```python
from build123d import *

# Parameters (mm, degrees)
F1_DEPTH = 5
F2_SIZE  = 2
F0_W     = 2.8
F0_H     = 9.8
F3_DEPTH = 2


# Not quite as in the source:
# - a feature of the source that left no trace in its solid (it failed there, or was rolled back) is left out


with BuildPart() as f1:
    # F0 (on Top) → F1 (new body)
    with BuildSketch(Plane.XY):
        Polygon((49.7136654785, 23.7398390386), (-80.2863345215, 29.3157004521), (-80.2863345215, 19.5157004521), (-80.2863345215, 15.7984595098), (49.7136654785, 15.7984595098), (73.3425258757, -14.2773987355), (73.3425258757, -14.4394316876), (85.7469019117, -14.4394316876), (88.3425258757, -11.6024324968), align=None)
    extrude(amount=F1_DEPTH)

    # F2 (call 1 of 5: OpenCascade refuses the feature's edges together)
    f2_edges = [f1.edges().sort_by_distance(p)[0] for p in [
        (-15.286335, 15.79846, 0),
    ]]
    chamfer(f2_edges, length=F2_SIZE)

    # F2#2 (call 2 of 5)
    f2_2_edges = [f1.edges().sort_by_distance(p)[0] for p in [
        (69.028096, 6.068703, 0),
    ]]
    chamfer(f2_2_edges, length=F2_SIZE)

    # F2#3 (call 3 of 5)
    f2_3_edges = [f1.edges().sort_by_distance(p)[0] for p in [
        (79.544714, -14.439432, 0),
    ]]
    chamfer(f2_3_edges, length=F2_SIZE)

    # F2#4 (call 4 of 5)
    f2_4_edges = [f1.edges().sort_by_distance(p)[0] for p in [
        (61.528096, 0.76053, 5),
        (-15.286335, 15.79846, 5),
    ]]
    chamfer(f2_4_edges, length=F2_SIZE)

    # F2#5 (call 5 of 5)
    f2_5_edges = [f1.edges().sort_by_distance(p)[0] for p in [
        (-15.286335, 26.52777, 5),
    ]]
    chamfer(f2_5_edges, length=F2_SIZE)

    # F0 (on Top) → F3 (join)
    with BuildSketch(Plane.XY):
        with Locations((-81.6863345215, 24.4157004521)):
            Rectangle(F0_W, F0_H)
    extrude(amount=F3_DEPTH)


solid = f1.part
```
Verification items for the finished model (mm, model axes). A direction names the side the tool comes from. Coordinates: 2 decimals unless noted, no trailing zeros. Loops run counter-clockwise (first coordinate to the right, second up) from the corner with the lowest first, then second, coordinate; pieces in that order, holes last. Notation, with made-up numbers: (-21.75, 11.25) - (-7.75, 11.25) arc R13 cw to (-7.75, 31.25) - close; hole circle Ø3 at (32.5, 88.25). An arc over 180 degrees is marked (long way). Put each result on its own line as item: value.
Item 1: Section check B-B (y = -7). Enter the section's corners in (x, z).
Conclusion:
outline: (67.63, 0) - (80.35, 0) - (83.31, 2) - (83.31, 5) - (70.17, 5) - (67.63, 3) - close
Item 2: Set-up check for faces 4 (the face through (73.343, -13, 4)), 5 (the face through (-14.38, 26.49, 1.48)), 6 (the face through (-82, 24, 2)): record each of +Z, -Z, +X, -X, +Y, -Y from which the full face is reachable in a straight line by a thin tool's end or side.
Conclusion:
face 4: +Z, -X, -Y
face 5: +Z, -Z, +X, +Y
face 6: +Z, -X, +Y, -Y
Item 3: Draft check along X on faces 1 (the face through (79, -14.439, 3)), 2 (the face through (69.3, 5.82, 3.48)), 3 (the face through (61.834, 1.968, 3.986)). Enter one of: pulls with the +X half, pulls with the -X half, needs draft (parallel to the pull), parting line crosses it, or undercut.
Conclusion:
face 1: needs draft
face 2: pulls with the +X half
face 3: pulls with the -X half
Item 4: Section check C-C (y = 4). Enter the section's corners in (x, z), then the cut area to 3 significant figures.
Conclusion:
outline: (58.98, 0) - (68.33, 0) - (71.29, 2) - (71.29, 5) - (61.53, 5) - (58.98, 3) - close
area: 56.0 mm2
Item 5: Scan lines: line 1 along Y through (x, z) = (38.5, 4.8); line 2 along Y through (x, z) = (-4, 1.25); line 3 along X through (y, z) = (23, 2.6). Record each from-to range of solid material in increasing order.
Conclusion:
line 1: y = 17.6 to 22.42
line 2: y = 16.55 to 26.04
line 3: x = -80.29 to 50.52
Item 6: Section check A-A (x = -42.5). Enter the section's corners in (y, z) (3 decimals), then the cut area to 3 significant figures.
Conclusion:
outline: (15.798, 2) - (17.798, 0) - (27.695, 0) - (27.695, 3) - (25.693, 5) - (17.798, 5) - (15.798, 3) - close
area: 53.5 mm2
Item 7: Section check D-D (x = 21). Enter the section's corners in (y, z), then the cut area to 3 significant figures.
Conclusion:
outline: (15.8, 2) - (17.8, 0) - (24.97, 0) - (24.97, 3) - (22.97, 5) - (17.8, 5) - (15.8, 3) - close
area: 39.9 mm2
Item 8: Gauge pin test, flat ends, axial feed: pin 1 Ø4 at (x, y) = (2.5, 13.5) entering from -Z; pin 2 Ø3 at (y, z) = (13.5, 3.5) entering from -X; pin 3 Ø1.6 at (x, z) = (-82.5, 1) entering from -Y; pin 4 Ø2 at (y, z) = (10, 1.5) entering from +X. Record the tip position at first contact, or that the pin passes through.
Conclusion:
pin 1: passes through
pin 2: stops at x = 50.41
pin 3: stops at y = 19.52
pin 4: stops at x = 65.68
